Print and shaded views of the part. All mm, measured from the part's lowest x, y and z. A direction names the side the tool comes from. Round coordinates to 2 decimals unless told otherwise and drop trailing zeros. Loops run counter-clockwise (first coordinate to the right, second up) from the corner with the lowest first, then second, coordinate; pieces in that order, holes last. Notation, with made-up numbers: (-22.5, -8) -> (17.5, -8) arc R25 ccw to (17.5, 10) -> close; hole circle Ø6 at (-29.5, 14). An arc over 180 degrees is marked (long way). Use a Markdown table: item, result.
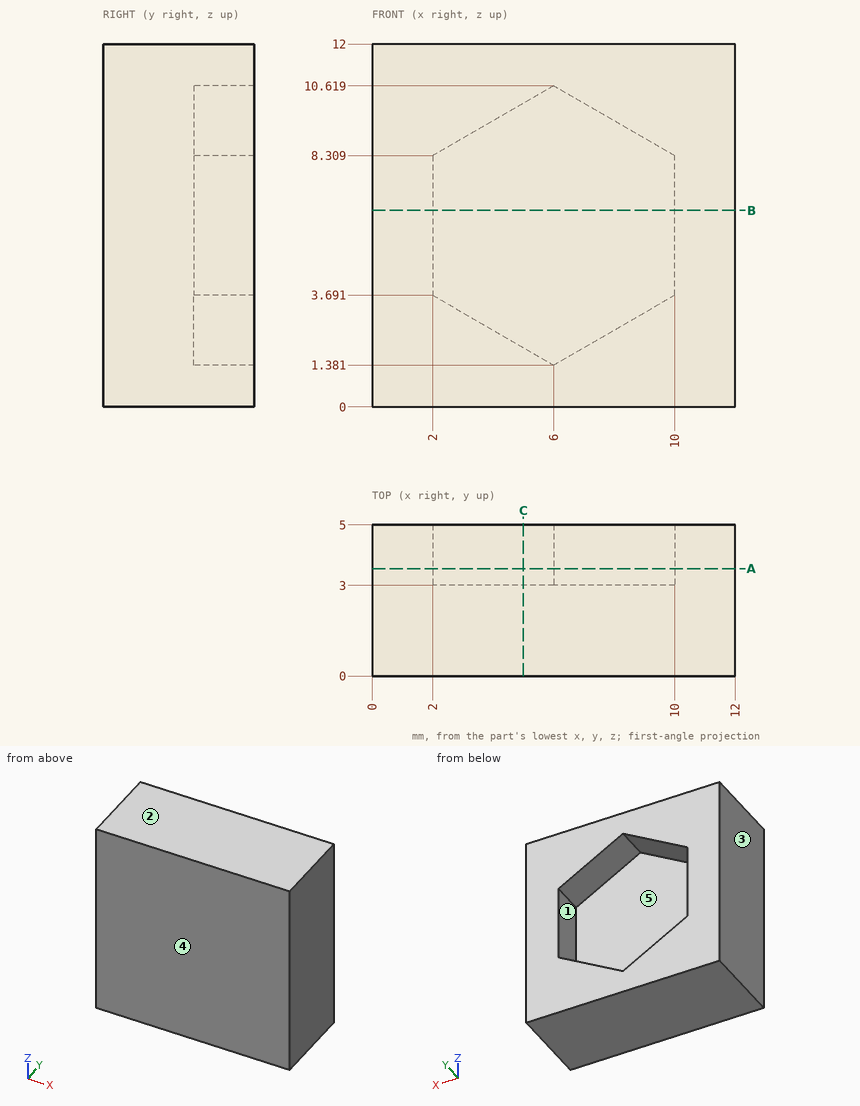
Q1. Drill centre lines: L1, parallel to X at y = 4.55, z = 4.5; L2, parallel to Y at x = 2.25, z = 5.75; L3, parallel to Z at x = 9.5, y = 4.8. Where is each one in solid material? Low to high. Write a range as from..to.
Results list:
| item | result |
|---|---|
| L1 | x = 0..2, 10..12 |
| L2 | y = 0..3 |
| L3 | z = 0..3.4, 8.6..12 |
Q2. Pull direction Z, two halves, no side cores. Call the marked faces 1, 2 and 3: released by +Z, released by -Z, zero draft, split by the parting line, or undercut.
Results list:
| item | result |
|---|---|
| face 1 | undercut |
| face 2 | released by +Z |
| face 3 | zero draft |
Q3. Band-saw the part on B-B, the plane z = 6.5. Give the cut face in (x, y), plus the area to 3 significant figures.
Results list:
| item | result |
|---|---|
| outline | (0, 0) -> (12, 0) -> (12, 5) -> (10, 5) -> (10, 3) -> (2, 3) -> (2, 5) -> (0, 5) -> close |
| area | 44.0 mm² |
Q4. Tool access for the marked faces 4 and 5: list every direction of +Z, -Z, +X, -X, +Y, -Y with a clear straight run to the whole face (end or side of a thin tool).
Results list:
| item | result |
|---|---|
| face 4 | +Z, -Z, +X, -X, -Y |
| face 5 | +Y |
Q5. Band-saw the part on A-A, the plane y = 3.55. Give the cut face in (x, z).
Results list:
| item | result |
|---|---|
| outline | (0, 0) -> (12, 0) -> (12, 12) -> (0, 12) -> close; hole (2, 3.69) -> (6, 1.38) -> (10, 3.69) -> (10, 8.31) -> (6, 10.62) -> (2, 8.31) -> close |
Q6. Band-saw the part on C-C, the plane x = 5. Give the cut face in (y, z).
Results list:
| item | result |
|---|---|
| outline | (0, 0) -> (5, 0) -> (5, 1.96) -> (3, 1.96) -> (3, 10.04) -> (5, 10.04) -> (5, 12) -> (0, 12) -> close |
Q7. Flat gauge pins, fed straight in: pin 1 (1.5 mm diameter, centred on x = 8.5, z = 4, fed in from -Y); pin 2 (2.5 mm diameter, centred on x = 8, z = 7, fed in from +Y). Where does each tip first touch, or does it go through?
Results list:
| item | result |
|---|---|
| pin 1 | stops at y = 0 |
| pin 2 | stops at y = 3 |
